Geometry: see drawing. Coordinates: mm, zero at the bounding-box minimum. A direction names the side the tool comes from. Coordinates: 2 decimals unless noted, no trailing zeros. Write each loop counter-clockwise with the first axis right and the second up, starting at its lowest first coordinate (ties: lowest second). Pieces come first, ordered by that corner, then holes. Notation, with made-up numbers: (-17, -27.5) - (16, -27.5) arc R21 cw to (16, 1.5) - close; hole circle Ø2 at (-35, -18.5). An arc over 180 degrees is marked (long way). Use CSV: the item, a comma, the result in double quotes.
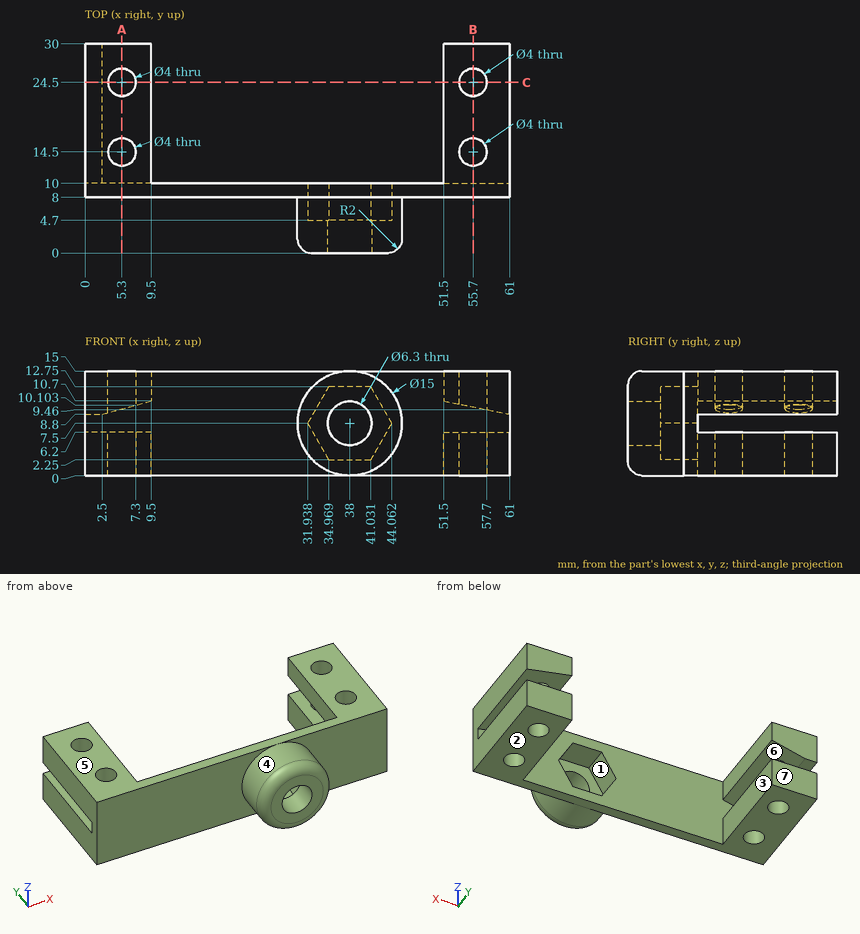
(1) Cut plane C-C on y = 24.5. State how many separate pieces and enclosed holes the cut face has, and give its area (3 significant figures).
Check values:
separate pieces,"8"
enclosed holes,"0"
area,"128 mm^2"
(2) Cut plane A-A on x = 5.3. Return loops of the section in (y, z).
Check values:
outline,"(8, 0) - (12.5, 0) - (12.5, 6.2) - (10, 6.2) - (10, 9.56) - (12.5, 9.56) - (12.5, 15) - (8, 15) - close; (16.5, 0) - (22.5, 0) - (22.5, 6.2) - (16.5, 6.2) - close; (16.5, 9.56) - (22.5, 9.56) - (22.5, 15) - (16.5, 15) - close; (26.5, 0) - (30, 0) - (30, 6.2) - (26.5, 6.2) - close; (26.5, 9.56) - (30, 9.56) - (30, 15) - (26.5, 15) - close"
(3) Draft query along Z for the marked faces 4, 5, 6 and 7. Return one class per face: pulls with the +Z half, pulls with the -Z half, needs draft (parallel to the pull), parting line crosses it, or undercut.
Check values:
face 4,"parting line crosses it"
face 5,"pulls with the +Z half"
face 6,"undercut"
face 7,"needs draft"
(4) Ray query, probe 1 along X at (y, z) = (14.5, 12); probe 2 along Y at (x, z) = (55.7, 4); probe 3 along X at (y, z) = (21.5, 14). Return the intervals inside material, ascending. Write a range as from..to.
Check values:
probe 1,"0..3.3, 7.3..9.5, 51.5..53.7, 57.7..61"
probe 2,"8..12.5, 16.5..22.5, 26.5..30"
probe 3,"0..9.5, 51.5..61"
(5) Reachability of the marked faces 1, 2 and 3 from +Z, -Z, +X, -X, +Y, -Y: full face, straight path, thin tool, end or side. Return the list, or none.
Check values:
face 1,"+Y"
face 2,"-Z, +X, -X, +Y, -Y"
face 3,"+Z, -Z, +Y"
(6) Pin query (flat end, axial travel): pin 1 Ø6 at (x, z) = (18, 3.5) entering from +Y; pin 2 Ø2.5 at (x, y) = (55.7, 24.5) entering from -Z; pin 3 Ø5 at (x, z) = (37.5, 5.5) entering from +Y. Return the tip coordinate at first contact, or that it passes through.
Check values:
pin 1,"y = 10"
pin 2,"through"
pin 3,"y = 4.7"
(7) Cut plane B-B on x = 55.7. Return loops of the section in (y, z).
Check values:
outline,"(8, 0) - (12.5, 0) - (12.5, 6.2) - (10, 6.2) - (10, 9.86) - (12.5, 9.86) - (12.5, 15) - (8, 15) - close; (16.5, 0) - (22.5, 0) - (22.5, 6.2) - (16.5, 6.2) - close; (16.5, 9.86) - (22.5, 9.86) - (22.5, 15) - (16.5, 15) - close; (26.5, 0) - (30, 0) - (30, 6.2) - (26.5, 6.2) - close; (26.5, 9.86) - (30, 9.86) - (30, 15) - (26.5, 15) - close"
